Read the model definition and answer for the solid it produces. Units are mm, in the model's axes. Coordinates: 2 decimals unless noted, no trailing zeros. Write each loop counter-clockwise with the first axis right and the second up, starting at its lowest first coordinate (ties: lowest second). Pieces come first, ordered by that corner, then holes. Notation, with made-up numbers: (-9, 42.5) -> (42, 42.5) arc R12 cw to (42, 60.5) -> close; hole circle Ø10 at (44, 71). An arc over 180 degrees is marked (long way). Answer in a Markdown table with one row per item. Add a question column.
Item 1: Straight lines are drawn through the part: line 1 (Y direction, x = 22.5, z = 1.4) (3 decimals); line 2 (X direction, y = -68.55, z = 1.55) (3 decimals); line 3 (Y direction, x = -28.5, z = 0.25) (3 decimals). For each, find the intervals that lie inside material, in ascending order. Write a range as from..to.
Item 2: Section B-B on x = 32.5 is taken. Write down the section's boundary in (y, z) (3 decimals), then the cut area to 3 significant figures.
Item 3: Section C-C on y = -90.5 is taken. Write down the section's boundary in (x, z) (3 decimals), then the cut area to 3 significant figures.
Item 4: Given pin 1 Ø1 at (y, z) = (-116, 2) entering from +X; pin 2 Ø1 at (y, z) = (93.5, 2.5) entering from -X (3 decimals); pin 3 Ø2 at (x, y) = (14, -7) entering from -Z; pin 4 Ø1 at (x, z) = (-43.5, 2) entering from -Y, each flat-ended and moving along its own axis, determine where each tip first touches the part or whether it passes through.
Item 5: Section A-A on z = 2 is taken. Count the separate pieces of the cut face and the enclosed holes in it, then the cut area to 3 significant figures.
```python
from build123d import *

# Parameters (mm, degrees)
SKETCH1_W           = 90
SKETCH1_H           = 235
SKETCH1_W_2         = 38
SKETCH1_H_2         = 49.5
SKETCH1_W_3         = 17
SKETCH1_H_3         = 26
SKETCH1_W_4         = 0.938488567
SKETCH1_R           = 1.4
SKETCH1_W_5         = 23.15
SKETCH1_H_4         = 81
SKETCH1_W_6         = 27.85
SKETCH1_W_7         = 35.5
SKETCH1_H_5         = 15
BOSS_EXTRUDE2_DEPTH = 3.175
SKETCH4_W           = 3.175
SKETCH4_H           = 18.25
CUT_EXTRUDE2_DEPTH  = 3.175
CUT_EXTRUDE3_DEPTH  = 4.175


with BuildPart() as part:
    # Sketch1 → Boss-Extrude2 (new body)
    with BuildSketch(Plane.XY):
        Rectangle(SKETCH1_W, SKETCH1_H)
        Polygon((-4.325, -114.325), (-39.825, -114.325), (-39.825, -99.325), (-41.825, -99.325), (-41.825, -96.15), (41.825, -96.15), (41.825, -99.325), (39.825, -99.325), (39.825, -114.325), (4.325, -114.325), (4.325, -99.325), (-4.325, -99.325), align=None, mode=Mode.SUBTRACT)
        Polygon((17.675, -94.15), (-10.175, -94.15), (-40.825, -94.15), (-40.825, -7.05), (17.675, -7.05), (17.675, -13.15), (40.825, -13.15), (40.825, -94.15), align=None, mode=Mode.SUBTRACT)
        with Locations((-22.825, 82.5)):
            Rectangle(SKETCH1_W_2, SKETCH1_H_2, mode=Mode.SUBTRACT)
        Polygon((23.761826634, 14.5), (6.761826634, 14.5), (6.761826634, 40.5), (23.761826634, 40.5), (24.700315201, 40.5), (41.700315201, 40.5), (41.700315201, 14.5), (24.700315201, 14.5), align=None, mode=Mode.SUBTRACT)
        with Locations((22.825, 82.5)):
            Rectangle(SKETCH1_W_2, SKETCH1_H_2, mode=Mode.SUBTRACT)
        with Locations((-22.825, 82.5)):
            Rectangle(SKETCH1_W_2, SKETCH1_H_2)
        with Locations((22.825, 82.5)):
            Rectangle(SKETCH1_W_2, SKETCH1_H_2)
        with Locations((33.200315201, 27.5)):
            Rectangle(SKETCH1_W_3, SKETCH1_H_3)
        with Locations((15.261826634, 27.5)):
            Rectangle(SKETCH1_W_3, SKETCH1_H_3)
        with Locations((24.231070918, 27.5)):
            Rectangle(SKETCH1_W_4, SKETCH1_H_3)
        Polygon((-40.825, -94.15), (-10.175, -94.15), (-10.175, -13.15), (17.675, -13.15), (17.675, -7.05), (-40.825, -7.05), align=None)
        with Locations((-34.825, -10.55)):
            Circle(SKETCH1_R, mode=Mode.SUBTRACT)
        with Locations((14.175, -10.55)):
            Circle(SKETCH1_R, mode=Mode.SUBTRACT)
        with Locations((29.25, -53.65)):
            Rectangle(SKETCH1_W_5, SKETCH1_H_4)
        with Locations((37.325, -90.65)):
            Circle(SKETCH1_R, mode=Mode.SUBTRACT)
        with Locations((37.325, -19.53)):
            Circle(SKETCH1_R, mode=Mode.SUBTRACT)
        with Locations((3.75, -53.65)):
            Rectangle(SKETCH1_W_6, SKETCH1_H_4)
        with Locations((14.175, -68.55)):
            Circle(SKETCH1_R, mode=Mode.SUBTRACT)
        with Locations((-22.075, -106.825)):
            Rectangle(SKETCH1_W_7, SKETCH1_H_5)
        with Locations((22.075, -106.825)):
            Rectangle(SKETCH1_W_7, SKETCH1_H_5)
        Polygon((-41.825, -99.325), (-39.825, -99.325), (-4.325, -99.325), (4.325, -99.325), (39.825, -99.325), (41.825, -99.325), (41.825, -96.15), (-41.825, -96.15), align=None)
        with Locations((37.325, -19.53)):
            Circle(SKETCH1_R)
        with Locations((37.325, -90.65)):
            Circle(SKETCH1_R)
    extrude(amount=BOSS_EXTRUDE2_DEPTH)

    # Sketch4 → Cut-Extrude2 (cut)
    with BuildSketch(Plane.XY.offset(3.175)):
        Polygon((-41.825, 114.325), (-20.25, 114.325), (-20.25, 117.5), (-45, 117.5), (-45, 79), (-41.825, 79), align=None)
        Polygon((41.825, 114.325), (41.825, 79), (45, 79), (45, 117.5), (20.25, 117.5), (20.25, 114.325), align=None)
        with Locations((-43.4125, 29.375)):
            Rectangle(SKETCH4_W, SKETCH4_H)
        with Locations((-43.4125, -29.375)):
            Rectangle(SKETCH4_W, SKETCH4_H)
        Polygon((-20.25, -117.5), (-20.25, -114.325), (-41.825, -114.325), (-41.825, -79), (-45, -79), (-45, -117.5), align=None)
        Polygon((45, -79), (41.825, -79), (41.825, -114.325), (20.25, -114.325), (20.25, -117.5), (45, -117.5), align=None)
        with Locations((43.4125, -29.375)):
            Rectangle(SKETCH4_W, SKETCH4_H)
        with Locations((43.4125, 29.375)):
            Rectangle(SKETCH4_W, SKETCH4_H)
    extrude(amount=-CUT_EXTRUDE2_DEPTH, mode=Mode.SUBTRACT)

    # Sketch5 → Cut-Extrude3 (cut, through all)
    with BuildSketch(Plane(origin=(0, 0, 0), x_dir=(-1, 0, 0), z_dir=(0, 0, -1))):
        with BuildLine():
            Line((-22.5, 38.75), (-22.5, 36.25))
            Line((-22.5, 36.25), (-20, 36.25))
            ThreePointArc((-20, 36.25), (-20.732233047, 38.017766953), (-22.5, 38.75))
        make_face()
        with BuildLine():
            Line((-20, 36.25), (-22.5, 36.25))
            Line((-22.5, 36.25), (-22.5, 38.75))
            ThreePointArc((-22.5, 38.75), (-24.267766953, 34.482233047), (-20, 36.25))
        make_face()
        with BuildLine():
            ThreePointArc((22.5, 38.75), (20.732233047, 38.017766953), (20, 36.25))
            Line((20, 36.25), (22.5, 36.25))
            Line((22.5, 36.25), (22.5, 38.75))
        make_face()
        with BuildLine():
            Line((22.5, 36.25), (20, 36.25))
            ThreePointArc((20, 36.25), (22.5, 33.75), (25, 36.25))
            ThreePointArc((25, 36.25), (24.267766953, 38.017766953), (22.5, 38.75))
            Line((22.5, 38.75), (22.5, 36.25))
        make_face()
        with BuildLine():
            ThreePointArc((20, 81.25), (20.732233047, 79.482233047), (22.5, 78.75))
            Line((22.5, 78.75), (22.5, 81.25))
            Line((22.5, 81.25), (20, 81.25))
        make_face()
        with BuildLine():
            Line((22.5, 81.25), (22.5, 78.75))
            ThreePointArc((22.5, 78.75), (24.267766953, 79.482233047), (25, 81.25))
            ThreePointArc((25, 81.25), (22.5, 83.75), (20, 81.25))
            Line((20, 81.25), (22.5, 81.25))
        make_face()
        with BuildLine():
            ThreePointArc((-20, 81.25), (-24.267766953, 83.017766953), (-22.5, 78.75))
            Line((-22.5, 78.75), (-22.5, 81.25))
            Line((-22.5, 81.25), (-20, 81.25))
        make_face()
        with BuildLine():
            Line((-22.5, 81.25), (-22.5, 78.75))
            ThreePointArc((-22.5, 78.75), (-20.732233047, 79.482233047), (-20, 81.25))
            Line((-20, 81.25), (-22.5, 81.25))
        make_face()
    extrude(amount=-CUT_EXTRUDE3_DEPTH, mode=Mode.SUBTRACT)


solid = part.part
```
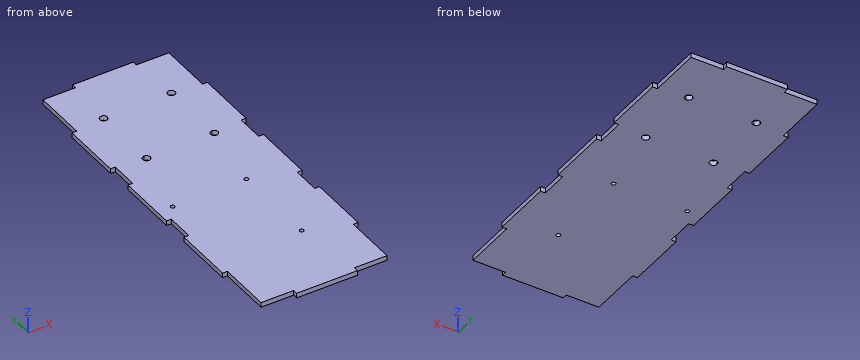
Results below:
| question | item | result |
|---|---|---|
| 1 | line 1 | y = -114.325..33.75, 38.75..78.75, 83.75..114.325 |
| 1 | line 2 | x = -45..12.775, 15.575..45 |
| 1 | line 3 | y = -114.325..114.325 |
| 2 | outline | (-114.325, 0) -> (114.325, 0) -> (114.325, 3.175) -> (-114.325, 3.175) -> close |
| 2 | area | 726 mm2 |
| 3 | outline | (-41.825, 0) -> (41.825, 0) -> (41.825, 3.175) -> (-41.825, 3.175) -> close |
| 3 | area | 266 mm2 |
| 4 | pin 1 | stops at x = 20.25 |
| 4 | pin 2 | stops at x = -41.825 |
| 4 | pin 3 | stops at z = 0 |
| 4 | pin 4 | stops at y = -79 |
| 5 | separate pieces | 1 |
| 5 | enclosed holes | 7 |
| 5 | area | 20,100 mm2 |
